Build history of the part. All positions in model axes, mm. Give positions to 0.01 mm unless a question says otherwise; leave off trailing zeros. Loops run counter-clockwise (first coordinate to the right, second up) from the corner with the lowest first, then second, coordinate; pieces in that order, holes last. Notation, with made-up numbers: (-38.75, 58.5) -> (-28.75, 58.5) arc R21 ccw to (-28.75, 74.5) -> close; hole circle Ø3 at (25.25, 11). An arc over 180 degrees is marked (long way). Answer as a JSON object with one key per item and string values. Group by question number.
from build123d import *

# Parameters (mm, degrees)
SKETCH1_W           = 50
SKETCH1_H           = 50
BOSS_EXTRUDE1_DEPTH = 8
HOLE1_D             = 6.3
HOLE1_CSINK_D       = 12
HOLE1_CSINK_ANGLE   = 90


with BuildPart() as part:
    # Sketch1 → Boss-Extrude1 (new body)
    with BuildSketch(Plane.XY):
        Rectangle(SKETCH1_W, SKETCH1_H)
    extrude(amount=BOSS_EXTRUDE1_DEPTH)

    # Hole1 (through all)
    with Locations(Plane(origin=(0, 12, 8), x_dir=(1, 0, 0), z_dir=(0, 0, 1))):
        with Locations((0, 0), (0, -24)):
            CounterSinkHole(HOLE1_D / 2, HOLE1_CSINK_D / 2, counter_sink_angle=HOLE1_CSINK_ANGLE)


solid = part.part
(1) Saw through at B-B on y = -12. List the corners of the cut face in (x, z), plus the area to 3 significant figures.
(2) Saw through at C-C on z = 3.75. List the corners of the cut face in (x, y), plus the area to 3 significant figures.
(3) Saw through at A-A on x = 0. List the corners of the cut face in (y, z).
(4) Pull direction Y, two halves, no side cores. Call faces 1 (the flat face through (-25, 0, 4)), 2 (the flat face through (0, -25, 4)), 3 (the cylindrical face through (0.41, 15.123, 2.539)), 4 (the cylindrical face through (0.41, -8.877, 2.539)): pulls with the +Y half, pulls with the -Y half, needs draft (parallel to the pull), parting line crosses it, or undercut.
(5) Pin check, flat tip, straight feed: pin 1 (3 mm diameter, centred on x = 15, y = 2, fed in from -Z). Stop position of the tip, or through.
(6) Probe line 1 along Y through (x, z) = (0, 3.8); line 2 along Y through (x, z) = (1, 4.5); line 3 along X through (y, z) = (12, 2.9). List the from-to ranges inside material, lowest first. Write a range as [from, to].
Calculated:
{
 "1": {"outline": "(-25, 0) -> (-3.15, 0) -> (-3.15, 5.15) -> (-6, 8) -> (-25, 8) -> close; (3.15, 0) -> (25, 0) -> (25, 8) -> (6, 8) -> (3.15, 5.15) -> close", "area": "341 mm^2"},
 "2": {"outline": "(-25, -25) -> (25, -25) -> (25, 25) -> (-25, 25) -> close; hole circle Ø6.3 at (0, -12); hole circle Ø6.3 at (0, 12)", "area": "2,440 mm^2"},
 "3": {"outline": "(-25, 0) -> (-15.15, 0) -> (-15.15, 5.15) -> (-18, 8) -> (-25, 8) -> close; (-8.85, 0) -> (8.85, 0) -> (8.85, 5.15) -> (6, 8) -> (-6, 8) -> (-8.85, 5.15) -> close; (15.15, 0) -> (25, 0) -> (25, 8) -> (18, 8) -> (15.15, 5.15) -> close"},
 "4": {"face 1": "needs draft", "face 2": "pulls with the -Y half", "face 3": "undercut", "face 4": "undercut"},
 "5": {"pin 1": "stops at z = 0"},
 "6": {"line 1": "y = [-25, -15.15], [-8.85, 8.85], [15.15, 25]", "line 2": "y = [-25, -14.99], [-9.01, 9.01], [14.99, 25]", "line 3": "x = [-25, -3.15], [3.15, 25]"}
}
